```python
from build123d import *
from build123d.topology import SkipClean

# Parameters (mm, degrees)
SKETCH1_W           = 40
SKETCH1_H           = 60
BOSS_EXTRUDE1_DEPTH = 10
SKETCH2_W           = 30
SKETCH2_H           = 40
BOSS_EXTRUDE2_DEPTH = 40
SKETCH6_R           = 15
SKETCH6_R_2         = 5
BOSS_EXTRUDE4_DEPTH = 20
SKETCH7_R           = 5
CUT_EXTRUDE2_DEPTH  = 30
CUT_EXTRUDE3_START  = 10
SKETCH8_W           = 30
SKETCH8_H           = 10
CUT_EXTRUDE3_DEPTH  = 50
BOSS_EXTRUDE5_START = 20
SKETCH10_R          = 3.25
BOSS_EXTRUDE5_DEPTH = 15
FILLET1_R           = 30
FILLET2_R           = 5
FILLET3_R           = 5
FILLET4_R           = 5
FILLET5_R           = 5
SCALE_1_SCALE       = 2
SKETCH_1_R          = 85
EXTRUDE_1_DEPTH     = 20
FILLET_1_R          = 10


# Some blends are built 0.0001 mm under size
with BuildPart() as part:
    # Sketch1 → Boss-Extrude1 (new body)
    with BuildSketch(Plane(origin=(0, 0, 0), x_dir=(1, 0, 0), z_dir=(0, 1, 0))):
        Rectangle(SKETCH1_W, SKETCH1_H)
    extrude(amount=BOSS_EXTRUDE1_DEPTH)

    # Sketch2 → Boss-Extrude2 (add)
    with BuildSketch(Plane(origin=(0, 0, 0), x_dir=(1, 0, 0), z_dir=(0, 1, 0))):
        Rectangle(SKETCH2_W, SKETCH2_H)
    extrude(amount=BOSS_EXTRUDE2_DEPTH)

    # Sketch6 → Boss-Extrude4 (add, symmetric)
    with BuildSketch(Plane.XY):
        with Locations((0, 40)):
            Circle(SKETCH6_R)
        with Locations((0, 40)):
            Circle(SKETCH6_R_2, mode=Mode.SUBTRACT)
    extrude(amount=BOSS_EXTRUDE4_DEPTH, both=True)

    # Sketch7 → Cut-Extrude2 (cut, symmetric)
    with SkipClean():  # the faces are left unmerged after this step: merging them gives an invalid solid
        with BuildSketch(Plane.XY):
            with Locations((0, 40)):
                Circle(SKETCH7_R)
        extrude(amount=CUT_EXTRUDE2_DEPTH, both=True, mode=Mode.SUBTRACT)

    # Sketch8 → Cut-Extrude3 (cut)
    with BuildSketch(Plane(origin=(0, 0, 0), x_dir=(1, 0, 0), z_dir=(0, 1, 0)).offset(CUT_EXTRUDE3_START)):
        Rectangle(SKETCH8_W, SKETCH8_H)
    extrude(amount=CUT_EXTRUDE3_DEPTH, mode=Mode.SUBTRACT)

    # Sketch10 → Boss-Extrude5 (add)
    with BuildSketch(Plane.XY.offset(BOSS_EXTRUDE5_START)):
        with BuildLine():
            Line((-49.142232779, 56.88315603), (-8.761443884, 27.824734045))
            ThreePointArc((-8.761443884, 27.824734045), (-12.990381057, 47.5), (6.163367673, 53.675265955))
            Line((6.163367673, 53.675265955), (-39.192358407, 74.11684397))
            ThreePointArc((-39.192358407, 74.11684397), (-51.961524227, 70), (-49.142232779, 56.88315603))
        make_face()
        with Locations((-43.301270189, 65)):
            Circle(SKETCH10_R, mode=Mode.SUBTRACT)
    extrude(amount=-BOSS_EXTRUDE5_DEPTH)

    # Fillet1
    fillet1_edges = [part.edges().sort_by_distance(p)[0] for p in [
        (-15, 32.314061796, 12.5),
    ]]
    fillet(fillet1_edges, radius=FILLET1_R)

    # Fillet2
    fillet2_edges = [part.edges().sort_by_distance(p)[0] for p in [
        (-38.309672505, 49.087936664, 20),
        (-38.309672505, 49.087936664, 5),
        (-18.300874237, 30.622707436, 5),
        (-18.300874237, 30.622707436, 20),
        (15, 25, 20),
        (12.598621256, 48.140930073, 20),
        (15, 25, 5),
        (12.598621256, 48.140930073, 5),
        (-51.961524227, 70, 20),
        (-16.514495367, 63.896054962, 5),
        (-51.961524227, 70, 5),
        (-16.514495367, 63.896054962, 20),
        (-15, 13.471092695, 20),
        (-15, 13.471092695, 5),
    ]]
    fillet(fillet2_edges, radius=FILLET2_R)

    # Fillet3
    fillet3_edges = [part.edges().sort_by_distance(p)[0] for p in [
        (15, 25, -20),
        (-15, 25, -20),
        (0, 55, -20),
        (-15, 25, -5),
        (0, 55, -5),
        (15, 25, -5),
    ]]
    fillet(fillet3_edges, radius=FILLET3_R)

    # Fillet4
    fillet4_edges = [part.edges().sort_by_distance(p)[0] for p in [
        (-20, 10, 0),
        (0, 10, 30),
        (20, 10, 0),
        (0, 10, -30),
    ]]
    fillet(fillet4_edges, radius=FILLET4_R - 0.0001)  # a hair under: the kernel refuses the full size

    # Fillet5
    # the kernel refuses this fillet: 5 mm, written as the material it takes off along each edge
    with BuildSketch(Plane(origin=(15, 10, 25), x_dir=(0, 0, 1), z_dir=(-1, 0, 0))) as fillet5_piece_1:
        with BuildLine():
            CenterArc((0.0001, -4.9999), 4.9999, 0, 90)
            Line((5, -4.9999), (5, 0))
            Line((5, 0), (0.0001, 0))
        make_face()
    revolve(axis=Axis((15, 10, 25), (0, 1, 0)), revolution_arc=90, mode=Mode.SUBTRACT)
    with BuildSketch(Plane(origin=(-15, 10, 25), x_dir=(-1, 0, 0), z_dir=(0, 0, -1))) as fillet5_piece_2:
        with BuildLine():
            CenterArc((0.0001, -4.9999), 4.9999, 0, 90)
            Line((5, -4.9999), (5, 0))
            Line((5, 0), (0.0001, 0))
        make_face()
    revolve(axis=Axis((-15, 10, 25), (0, 1, 0)), revolution_arc=90, mode=Mode.SUBTRACT)
    with BuildSketch(Plane(origin=(15, 10, -25), x_dir=(1, 0, 0), z_dir=(0, 0, 1))) as fillet5_piece_3:
        with BuildLine():
            CenterArc((0.0001, -4.9999), 4.9999, 0, 90)
            Line((5, -4.9999), (5, 0))
            Line((5, 0), (0.0001, 0))
        make_face()
    revolve(axis=Axis((15, 10, -25), (0, 1, 0)), revolution_arc=90, mode=Mode.SUBTRACT)
    with BuildSketch(Plane(origin=(-15, 10, -25), x_dir=(0, 0, -1), z_dir=(1, 0, 0))) as fillet5_piece_4:
        with BuildLine():
            CenterArc((0.0001, -4.9999), 4.9999, 0, 90)
            Line((5, -4.9999), (5, 0))
            Line((5, 0), (0.0001, 0))
        make_face()
    revolve(axis=Axis((-15, 10, -25), (0, 1, 0)), revolution_arc=90, mode=Mode.SUBTRACT)
    with BuildSketch(Plane(origin=(-20, -12.5, -30), x_dir=(0, 0, 1), z_dir=(0, 1, 0)), Plane(origin=(20, -12.5, -30), x_dir=(-1, 0, 0), z_dir=(0, 1, 0))) as fillet5_piece_5:
        with BuildLine():
            CenterArc((FILLET5_R, FILLET5_R), FILLET5_R, 180, 90)
            Line((0, FILLET5_R), (0, 0))
            Line((0, 0), (FILLET5_R, 0))
        make_face()
    extrude(amount=22.5, mode=Mode.SUBTRACT)
    with BuildSketch(Plane(origin=(20, -12.5, 30), x_dir=(-1, 0, 0), z_dir=(0, 1, 0)), Plane(origin=(-20, -12.5, 30), x_dir=(0, 0, -1), z_dir=(0, 1, 0))) as fillet5_piece_6:
        with BuildLine():
            CenterArc((FILLET5_R, -FILLET5_R), FILLET5_R, 90, 90)
            Line((0, -FILLET5_R), (0, 0))
            Line((0, 0), (FILLET5_R, 0))
        make_face()
    extrude(amount=22.5, mode=Mode.SUBTRACT)


with BuildPart() as part_1:
    # 缩放比例1: scaled about (-5.855669763, 27.313859585, 2.636754643)
    add(part.part.scale(SCALE_1_SCALE).moved(Location((5.855669763, -27.313859585, -2.636754643))))

    # 草图1 → 凸台-拉伸1 (add)
    with BuildSketch(Plane.XZ.offset(27.313870031)):
        with Locations(Location((5.855672976, -2.63675609, 0), (0, 0, 270))):
            Circle(SKETCH_1_R)
    extrude(amount=-EXTRUDE_1_DEPTH)

    # 圆角1
    fillet_1_edges = [part_1.edges().sort_by_distance(p)[0] for p in [
        (5.855672976, -7.313870031, 82.36324391),
    ]]
    fillet(fillet_1_edges, radius=FILLET_1_R)


solid = part_1.part
```
Can you work these out from the model? Positions are in its coordinate system, mm. A direction names the side the tool comes from. Round coordinates to 2 decimals unless told otherwise and drop trailing zeros. One line per item, written item: value. Start each with the question number.
1. If we section it at A-A, the plane y = 46.5: Give the number of separate pieces and of enclosed holes in the cut face, then the cut area to 3 significant figures.
2. For faces 1 (the flat face through (-20, 54, 37.363)), 2 (the cylindrical face through (-68.795, 72.958, 10.37)), 3 (the cylindrical face through (-30.929, 34.285, 22.433)), 4 (the cylindrical face through (33, 23.11, 34.36)), 5 (the cylindrical face through (-68.79, 72.96, 34.36)), which set-ups out of +Z, -Z, +X, -X, +Y, -Y let a thin tool reach every point of the face, with its end or its side?
3. If we mould it in two halves opening along Y, with no side actions, what happens to faces 6 (the flat face through (7, -27.314, -1)), 7 (the cylindrical face through (11.23, 61.12, 22.15)), 8 (the flat face through (-24.144, 22, -28)), 9 (the cylindrical face through (31.18, 68.77, 22.43))? For each: pulls with the +Y half, pulls with the -Y half, needs draft (parallel to the pull), parting line crosses it, or undercut.
4. If I drill on probe 1 along Z at (x, y) = (-1.5, -7); probe 2 along Y at (x, z) = (-14.5, 67.5); probe 3 along X at (y, z) = (61, 21.5), over which ranges is the centre line in solid material (lowest first)?
5. For pin 1 (2 mm diameter, centred on x = -41.5, y = 62, fed in from -Z); pin 2 (16 mm diameter, centred on x = 5.86, y = 52.69, fed in from -Z); pin 3 (21 mm diameter, centred on x = -80.75, y = 102.69, fed in from +Z); pin 4 (5 mm diameter, centred on y = 58.5, z = 18, fed in from -X), each with a flat end and sliding along its axis, tell me the tip position at first contact or that it passes through.
Calculated:
1. separate pieces: 4
1. enclosed holes: 0
1. area: 2,930 mm²
2. face 1: +Z, +X, -X, +Y
2. face 2: -Z, -X
2. face 3: +Z, -Z, -X
2. face 4: +Z, +X, +Y
2. face 5: +Z, -X
3. face 6: pulls with the -Y half
3. face 7: undercut
3. face 8: needs draft
3. face 9: pulls with the +Y half
4. probe 1: z = -42.64 to -12.64, 7.36 to 37.36
4. probe 2: y = -27.31 to -7.31
4. probe 3: x = -57.06 to 0.3, 11.41 to 34.68
5. pin 1: stops at z = 7.36
5. pin 2: passes through
5. pin 3: stops at z = 37.36
5. pin 4: stops at x = -57.06
